Answer from the drawing. Dimensions are ordinates in mm from the lowest x, y and z of the part. A direction names the side the tool comes from. Coordinates: 2 decimals unless noted, no trailing zeros. Write each loop counter-clockwise with the first axis right and the second up, starting at its lowest first coordinate (ties: lowest second). Pieces come first, ordered by that corner, then holes. Notation, with made-up numbers: M 9,59.25 L 59,59.25 A19 ccw 59,91.25 Z; hole C -2,14 d10. An arc over 180 degrees is marked long. Put each result on its own line as item: value. Start each with the question number.
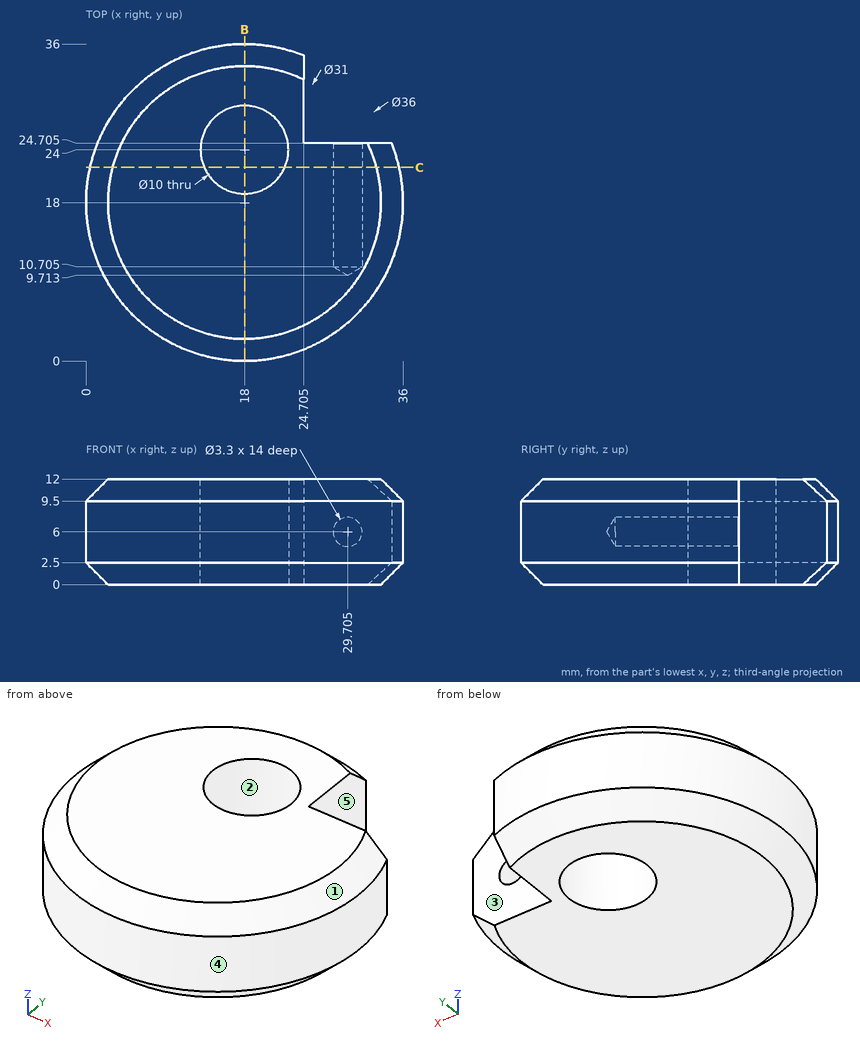
1) A cutting plane is placed at B-B on x = 18. Write down the section's boundary in (y, z).
2) Given pin 1 Ø3 at (y, z) = (21.5, 6) entering from -X; pin 2 Ø4.5 at (x, z) = (29.7, 6) entering from -Y; pin 3 Ø5 at (x, z) = (8, 4.5) entering from -Y, each flat-ended and moving along its own axis, determine where each tip first touches the part or whether it passes through.
3) A cutting plane is placed at C-C on y = 22. State how many separate pieces and enclosed holes the cut face has, then the cut area to 3 significant figures.
4) For the marked faces 4 and 5, determine the directions among +Z, -Z, +X, -X, +Y, -Y from which every point of the face is accessible in a straight line to the end or side of a thin tool.
5) Determine the mould class of the marked faces 1, 2 and 3 for opening direction X: +X half, -X half, draft (parallel to the pull), parting line (faces both ways), or undercut.
6) Straight lines are drawn through the part: probe 1 along Y at (x, z) = (18, 5.25); probe 2 along X at (y, z) = (20.5, 6) (1 decimal); probe 3 along Y at (x, z) = (15.5, 11). For each, find the intervals that lie inside material, in ascending order.
Answers follow:
1. outline: M 0,2.5 L 2.5,0 L 19,0 L 19,12 L 2.5,12 L 0,9.5 Z; M 29,0 L 33.5,0 L 36,2.5 L 36,9.5 L 33.5,12 L 29,12 Z
2. pin 1: stops at x = 0.11
2. pin 2: stops at y = 2.68
2. pin 3: stops at y = 1.64
3. separate pieces: 2
3. enclosed holes: 1
3. area: 290 mm²
4. face 4: +Z, -Z
4. face 5: +Z, -Z, +X, +Y
5. face 1: parting line
5. face 2: undercut
5. face 3: draft
6. probe 1: y = 0 to 19, 29 to 36
6. probe 2: x = 0.2 to 14.4, 21.6 to 28.1, 31.4 to 35.8
6. probe 3: y = 1.69 to 19.67, 28.33 to 34.31
